from build123d import *

# Parameters (mm, degrees)
SKETCH_1_W        = 5
SKETCH_1_H        = 5
EXTRUDE_2_DEPTH   = 165
EXTRUDE_2_2_DEPTH = 165
SKETCH_2_R        = 2.5
EXTRUDE_3_DEPTH   = 27


with BuildPart() as part:
    # Sketch 1 → Extrude 2 (new body)
    with BuildSketch(Plane(origin=(0, 0, 0), x_dir=(1, 0, 0), z_dir=(0, 1, 0))):
        with Locations((-18.035714286, 2.5)):
            Rectangle(SKETCH_1_W, SKETCH_1_H)
    extrude(amount=-EXTRUDE_2_DEPTH)



with BuildPart() as body_2:
    # Sketch 1 → Extrude 2 2 (new body)
    with BuildSketch(Plane(origin=(0, 0, 0), x_dir=(1, 0, 0), z_dir=(0, 1, 0))):
        with Locations((13.964285714, 2.5)):
            Rectangle(SKETCH_1_W, SKETCH_1_H)
    extrude(amount=-EXTRUDE_2_2_DEPTH)


with BuildPart() as part_1:
    add(part.part)

    add(body_2.part)  # Extrude 3 merges body 2
    # Sketch 2 → Extrude 3 (add)
    with BuildSketch(Plane(origin=(-15.535714286, 0, 0), x_dir=(0, 0, -1), z_dir=(1, 0, 0))):
        with Locations(Location((2.5, -162.5, 0), (0, 0, 180))):
            Circle(SKETCH_2_R)
        with Locations(Location((2.5, -155.5, 0), (0, 0, 180))):
            Circle(SKETCH_2_R)
    extrude(amount=EXTRUDE_3_DEPTH)


solid = part_1.part
Geometry check sheet. Reference: the model listing, model coordinates, mm. A direction names the side the tool comes from. Give positions to 0.01 mm unless a question says otherwise; leave off trailing zeros. Loops run counter-clockwise (first coordinate to the right, second up) from the corner with the lowest first, then second, coordinate; pieces in that order, holes last.
(1) Thickness scan on L1, parallel to X at y = -133.5, z = -1; L2, parallel to Y at x = -10.5, z = -2.65; L3, parallel to Y at x = 1, z = -1.75. Record the ranges inside material, lowest first.
From the geometry:
L1: x = -20.54 to -15.54, 11.46 to 16.46
L2: y = -165 to -160, -158 to -153
L3: y = -164.88 to -160.12, -157.88 to -153.12
(2) Release check for a two-part mould opening along Y. For faces 3 (the flat face through (11.464, -159, -2)), 4 (the flat face through (14, -165, -3)), 5 (the flat face through (-18, -81, 0)), 6 (the cylindrical face through (-2.22, -164.98, -2.83)) record: released by +Y, released by -Y, zero draft, split by the parting line, or undercut.
From the geometry:
face 3: undercut
face 4: released by -Y
face 5: zero draft
face 6: undercut
(3) Section check A-A on y = -40.5. Record the cut outline in (x, z), then the cut area to 3 significant figures.
From the geometry:
outline: (-20.54, -5) - (-15.54, -5) - (-15.54, 0) - (-20.54, 0) - close; (11.46, -5) - (16.46, -5) - (16.46, 0) - (11.46, 0) - close
area: 50.0 mm2
(4) Set-up check for faces 1 (the cylindrical face through (-2.22, -157.98, -2.83)), 2 (the flat face through (14, -81, -5)): record each of +Z, -Z, +X, -X, +Y, -Y from which the full face is reachable in a straight line by a thin tool's end or side.
From the geometry:
face 1: none
face 2: -Z, +X, -X, +Y, -Y
(5) Section check B-B on x = -1. Record the cut outline in (y, z).
From the geometry:
outline: circle Ø5 at (-162.5, -2.5); circle Ø5 at (-155.5, -2.5)
(6) Section check C-C on z = -3.6. Record the cut outline in (x, y) (3 decimals).
From the geometry:
outline: (-20.536, -165) - (-15.536, -165) - (-15.536, -164.745) - (11.464, -164.745) - (11.464, -165) - (16.464, -165) - (16.464, 0) - (11.464, 0) - (11.464, -153.255) - (-15.536, -153.255) - (-15.536, 0) - (-20.536, 0) - close; hole (-15.536, -160.255) - (11.464, -160.255) - (11.464, -157.745) - (-15.536, -157.745) - close
(7) Depth check by flat-ended pin: pin 1 Ø2 at (x, z) = (-3, -1) entering from -Y. Enter the tip coordinate at first touch or a pass-through.
From the geometry:
pin 1: stops at y = -164.95
